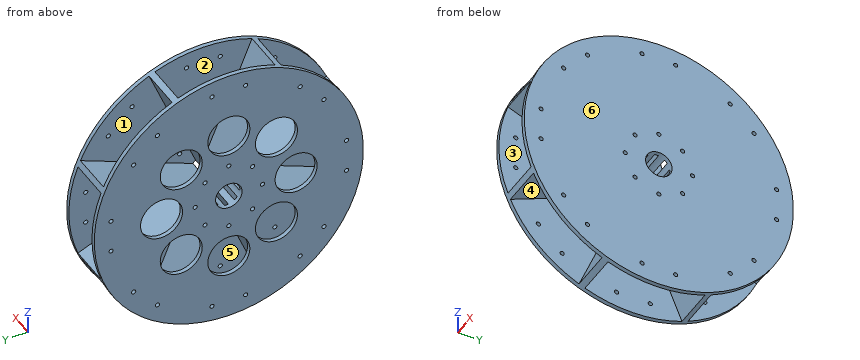
```python
from build123d import *

# Parameters (mm, degrees)
SKETCH1_R           = 203.2
BOSS_EXTRUDE1_DEPTH = 76.2
SKETCH6_R           = 31.75
SKETCH6_R_2         = 3.175
CUT_EXTRUDE1_DEPTH  = 298.299377732
CIRPATTERN1_COUNT   = 8
CUT_EXTRUDE3_DEPTH  = 31.75
CIRPATTERN2_COUNT   = 8
SKETCH11_R          = 31.75
BOSS_EXTRUDE2_DEPTH = 6.35
CIRPATTERN4_COUNT   = 8
CUT_EXTRUDE4_REACH  = 299.299
SKETCH12_R          = 20


with BuildPart() as part:
    # Sketch1 → Boss-Extrude1 (new body)
    with BuildSketch(Plane(origin=(0, 0, 0), x_dir=(0, 0, -1), z_dir=(1, 0, 0))):
        with Locations(Location((0, 0, 0), (0, 0, 180))):
            Circle(SKETCH1_R)
    extrude(amount=BOSS_EXTRUDE1_DEPTH)

    # Sketch6 → Cut-Extrude1 (cut, through all)
    with BuildSketch(Plane(origin=(76.2, 0, 0), x_dir=(0, 0, -1), z_dir=(1, 0, 0))):
        with Locations((0, 101.6)):
            Circle(SKETCH6_R)
        with Locations((25.4, 177.8)):
            Circle(SKETCH6_R_2)
        with Locations((-25.4, 177.8)):
            Circle(SKETCH6_R_2)
        with Locations((0, 50.8)):
            Circle(SKETCH6_R_2)
    cut_extrude1 = extrude(amount=-CUT_EXTRUDE1_DEPTH, mode=Mode.SUBTRACT)

    # CirPattern1: Cut-Extrude1 ×8 about axis
    cirpattern1_axis = Axis((0, 0, 0), (1, 0, 0))
    for i in range(1, CIRPATTERN1_COUNT):
        add(cut_extrude1.rotate(cirpattern1_axis, i * 360 / CIRPATTERN1_COUNT), mode=Mode.SUBTRACT)

    # Sketch8 → Cut-Extrude3 (cut, symmetric)
    with BuildSketch(Plane(origin=(38.1, 0, 0), x_dir=(0, 0, -1), z_dir=(1, 0, 0))):
        with BuildLine():
            Line((12.7, 0), (189.538488464, -73.248900271))
            ThreePointArc((189.538488464, -73.248900271), (203.2, 0), (189.538488464, 73.248900271))
            Line((189.538488464, 73.248900271), (12.7, 0))
        make_face()
    cut_extrude3 = extrude(amount=CUT_EXTRUDE3_DEPTH, both=True, mode=Mode.SUBTRACT)

    # CirPattern2: Cut-Extrude3 ×8 about axis
    cirpattern2_axis = Axis((0, 0, 0), (1, 0, 0))
    for i in range(1, CIRPATTERN2_COUNT):
        add(cut_extrude3.rotate(cirpattern2_axis, i * 360 / CIRPATTERN2_COUNT), mode=Mode.SUBTRACT)

    # Sketch11 → Boss-Extrude2 (add)
    with BuildSketch(Plane(origin=(76.2, 0, 0), x_dir=(0, 0, -1), z_dir=(1, 0, 0))):
        with Locations((0, 101.6)):
            Circle(SKETCH11_R)
    boss_extrude2 = extrude(amount=-BOSS_EXTRUDE2_DEPTH)

    # CirPattern4: Boss-Extrude2 ×8 about axis
    cirpattern4_axis = Axis((0, 0, 0), (-1, 0, 0))
    for i in range(1, CIRPATTERN4_COUNT):
        add(boss_extrude2.rotate(cirpattern4_axis, i * 360 / CIRPATTERN4_COUNT))

    # Cut-Extrude4: up to this face of the body (flat: up to its plane)
    cut_extrude4_end = Plane(part.part.faces().sort_by_distance((76.2, 0, 0))[0])
    # Sketch12 → Cut-Extrude4 (cut, up to the picked face)
    with BuildSketch(Plane.ZY, mode=Mode.PRIVATE) as cut_extrude4_sk1:
        Circle(SKETCH12_R)
    cut_extrude4_tool1 = split(extrude(cut_extrude4_sk1.sketch, amount=-CUT_EXTRUDE4_REACH, mode=Mode.PRIVATE), bisect_by=cut_extrude4_end, keep=Keep.BOTH, mode=Mode.PRIVATE)
    add(cut_extrude4_tool1.solids().sort_by(Axis((0, 0, 0), (1, 0, 0)))[0], mode=Mode.SUBTRACT)


solid = part.part
```
The listing builds one solid part. Answer for the finished solid, in the listing's coordinates (mm). Face numbers are marked on the shaded views. A direction names the side the tool comes from. Round coordinates to 2 decimals unless told otherwise and drop trailing zeros. Loops run counter-clockwise (first coordinate to the right, second up) from the corner with the lowest first, then second, coordinate; pieces in that order, holes last.
1) A cutting plane is placed at A-A on x = 25.5. Give the number of separate pieces and of enclosed holes in the cut face, plus the area to 3 significant figures.
Outcome:
separate pieces: 8
enclosed holes: 0
area: 14,300 mm2
2) Consider line 1 (Y direction, x = 2.25, z = 0) (3 decimals); line 2 (X direction, y = 101, z = -58); line 3 (Y direction, x = 46, z = -29). Determine where each line is inside the solid, lowest interval first.
Outcome:
line 1: y = -203.2 to -133.35, -69.85 to -53.975, -47.625 to -20, 20 to 47.625, 53.975 to 69.85, 133.35 to 203.2
line 2: x = 0 to 6.35, 69.85 to 76.2
line 3: y = -82.71 to -57.31, -17.27 to -6.75, 6.75 to 17.27, 57.31 to 82.71
3) For the marked faces 1, 2 and 3, determine the directions among +Z, -Z, +X, -X, +Y, -Y from which every point of the face is accessible in a straight line to the end or side of a thin tool.
Outcome:
face 1: none
face 2: +Z
face 3: -Y
4) A cutting plane is placed at D-D on y = 120.5. Determine the outline of the cut face in (x, z).
Outcome:
outline: (0, -163.62) - (6.35, -163.62) - (6.35, -55.17) - (69.85, -55.17) - (69.85, -163.62) - (76.2, -163.62) - (76.2, 163.62) - (69.85, 163.62) - (69.85, 55.17) - (6.35, 55.17) - (6.35, 163.62) - (0, 163.62) - (0, 25.51) - (6.35, 25.51) - (6.35, 44.65) - (69.85, 44.65) - (69.85, -44.65) - (6.35, -44.65) - (6.35, -25.51) - (0, -25.51) - close
5) A cutting plane is placed at C-C on z = -126.5. Determine the outline of the cut face in (x, y), plus the area to 3 significant figures.
Outcome:
outline: (0, -159.02) - (6.35, -159.02) - (6.35, -57.66) - (69.85, -57.66) - (69.85, -159.02) - (76.2, -159.02) - (76.2, 159.02) - (69.85, 159.02) - (69.85, 57.66) - (6.35, 57.66) - (6.35, 159.02) - (0, 159.02) - (0, 19.7) - (6.35, 19.7) - (6.35, 47.14) - (69.85, 47.14) - (69.85, -47.14) - (6.35, -47.14) - (6.35, -19.7) - (0, -19.7) - close
area: 5,130 mm2
6) Given P1, Ø5, axis at y = -50.8, z = 0, coming from the +X side; P2, Ø12, axis at x = 17, z = 5, coming from the -Y side; P3, Ø4, axis at x = 32.5, z = -40, coming from the -Y side; P4, Ø5, axis at x = 64.5, z = -77, coming from the -Y side, each flat-ended and moving along its own axis, determine where each tip first touches the part or whether it passes through.
Outcome:
P1: passes through
P2: stops at y = -39.26
P3: stops at y = -114.1
P4: stops at y = -189.05
7) For a pull along X with two mould halves and no side action, classify the marked faces 4, 5 and 6 as released by +X, released by -X, zero draft, split by the parting line, or undercut.
Outcome:
face 4: undercut
face 5: undercut
face 6: released by +X
